from build123d import *

# Parameters (mm, degrees)
BOSS_EXTRUDE1_DEPTH = 6
FILLET1_R           = 2


with BuildPart() as part:
    # Sketch1 → Boss-Extrude1 (new body)
    with BuildSketch(Plane.XY):
        with BuildLine():
            Line((4, 32.627416998), (8, 32.627416998))
            Line((8, 32.627416998), (8, 22.627416998))
            ThreePointArc((8, 22.627416998), (23.949344099, -1.558498392), (5, -23.473389189))
            Line((5, -23.473389189), (5, -31.473389189))
            Line((5, -31.473389189), (-5, -31.473389189))
            Line((-5, -31.473389189), (-5, -23.473389189))
            ThreePointArc((-5, -23.473389189), (-23.949344099, -1.558498392), (-8, 22.627416998))
            Line((-8, 22.627416998), (-8, 32.627416998))
            Line((-8, 32.627416998), (-4, 32.627416998))
            Line((-4, 32.627416998), (-4, 19.595917942))
            ThreePointArc((-4, 19.595917942), (0, -20), (4, 19.595917942))
            Line((4, 19.595917942), (4, 32.627416998))
        make_face()
    extrude(amount=BOSS_EXTRUDE1_DEPTH)

    # Fillet1
    fillet1_edges = [part.edges().sort_by_distance(p)[0] for p in [
        (-4, 19.595917942, 3),
        (4, 19.595917942, 3),
        (-8, 22.627416998, 3),
        (8, 32.627416998, 3),
        (4, 32.627416998, 3),
        (-4, 32.627416998, 3),
        (-8, 32.627416998, 3),
        (-5, -31.473389189, 3),
        (-5, -23.473389189, 3),
        (5, -31.473389189, 3),
        (5, -23.473389189, 3),
        (8, 22.627416998, 3),
    ]]
    fillet(fillet1_edges, radius=FILLET1_R - 0.0001)  # a hair under: the kernel refuses the full size


solid = part.part
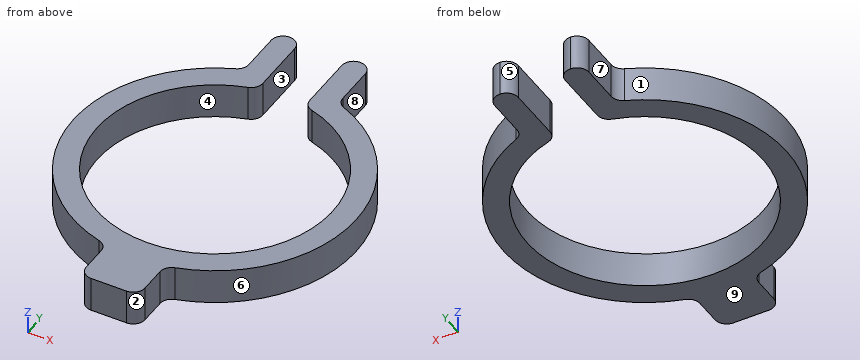
Geometry: final body of the model. Coordinates: model frame, mm. Face numbers are marked on the shaded views. A direction names the side the tool comes from. Round coordinates to 2 decimals unless told otherwise and drop trailing zeros. Loops run counter-clockwise (first coordinate to the right, second up) from the corner with the lowest first, then second, coordinate; pieces in that order, holes last.
Q1. Section A-A on y = 0. Return loops of the section in (x, z), plus the area to 3 significant figures.
Q2. Material intervals for L1, parallel to X at y = 0, z = 2.75; L2, parallel to Y at x = 0, z = 4.5; L3, parallel to Y at x = -11, z = 1.25, sorted ascending.
Q3. Pull-direction query (X, two-part tool) for the marked faces 1, 2, 3 and 4; classes: released by +X, released by -X, zero draft, split by the parting line, or undercut.
Q4. Access query for the marked faces 5, 6, 7, 8 and 9. Directions: +Z, -Z, +X, -X, +Y, -Y. A direction counts if a zero-diameter tool reaches every point of the face in a straight line with its end or side. Return the directions, or none.
Q5. Section C-C on x = 0. Return loops of the section in (y, z).
Q6. Section D-D on y = 9. Return loops of the section in (x, z).
Q7. Pin query (flat end, axial travel): P1, Ø1.5, axis at x = -15.5, z = 5.5, coming from the -Y side; P2, Ø24, axis at x = 0, y = 0, coming from the -Z side; P3, Ø2, axis at y = 18.5, z = 3.5, coming from the -X side; P4, Ø3, axis at y = 27.5, z = 3.5, coming from the -X side. Return the tip coordinate at first contact, or that it passes through.
Evaluation:
1. outline: (-24, 0) - (-20, 0) - (-20, 6) - (-24, 6) - close; (20, 0) - (24, 0) - (24, 6) - (20, 6) - close
1. area: 48.0 mm2
2. L1: x = -24 to -20, 20 to 24
2. L2: y = -31.47 to -20
2. L3: y = -21.33 to -16.7, 16.7 to 21.33
3. face 1: released by -X
3. face 2: released by +X
3. face 3: undercut
3. face 4: undercut
4. face 5: +Z, -Z, +Y
4. face 6: +Z, -Z, +X
4. face 7: +Z, -Z, -X, +Y
4. face 8: +Z, -Z, +X, +Y
4. face 9: -Z, +X, -X, +Y, -Y
5. outline: (-31.47, 0) - (-20, 0) - (-20, 6) - (-31.47, 6) - close
6. outline: (-22.25, 0) - (-17.86, 0) - (-17.86, 6) - (-22.25, 6) - close; (17.86, 0) - (22.25, 0) - (22.25, 6) - (17.86, 6) - close
7. P1: stops at y = -18.93
7. P2: passes through
7. P3: stops at x = -16.42
7. P4: stops at x = -8
